For this review, take the finished solid that the model builds, in its own axes (mm). A direction names the side the tool comes from. Round coordinates to 2 decimals unless told otherwise and drop trailing zeros. Order: outer loops, then holes, each group sorted by start corner. A loop starts at its lowest first (then second) coordinate and runs counter-clockwise, first axis right, second up. Notation, with made-up numbers: (-15, -31.5) -> (31, -31.5) arc R19 ccw to (31, 5.5) -> close; hole circle Ø7 at (35.25, 68.25). An arc over 180 degrees is marked (long way). Answer in a Markdown table with one row per item.
```python
from build123d import *

# Parameters (mm, degrees)
F0_W     = 15
F0_H     = 90
F0_R     = 1.5
F1_DEPTH = 3
F2_W     = 15
F2_H     = 3
F3_DEPTH = 18
F4_R     = 2.25
F5_DEPTH = 53.001


with BuildPart() as f1:
    # F0 (on Front) → F1 (new body)
    with BuildSketch(Plane.XZ):
        Rectangle(F0_W, F0_H)
        with Locations((0, -39)):
            Circle(F0_R, mode=Mode.SUBTRACT)
        with Locations((0, 41)):
            Circle(F0_R, mode=Mode.SUBTRACT)
    extrude(amount=F1_DEPTH)

    # F2 (on face) → F3 (join)
    with BuildSketch(Plane.XZ.offset(3)):
        with Locations((0, 6.5)):
            Rectangle(F2_W, F2_H)
    extrude(amount=F3_DEPTH)

    # F4 (on face) → F5 (cut, through all)
    with BuildSketch(Plane.XY.offset(8)):
        with Locations((0, -12)):
            Circle(F4_R)
    extrude(amount=-F5_DEPTH, mode=Mode.SUBTRACT)


solid = f1.part
```
Q1. To check wall thickness, follow probe 1 along Z at (x, y) = (0, -1.7); probe 2 along Y at (x, z) = (0, 7); probe 3 along Z at (x, y) = (1.5, -13.75). State the ranges of each line that lie inside material, in increasing order.
Answer key:
| item | result |
|---|---|
| probe 1 | z = -45 to -40.5, -37.5 to 39.5, 42.5 to 45 |
| probe 2 | y = -21 to -14.25, -9.75 to 0 |
| probe 3 | z = 5 to 8 |
Q2. Take a section at A-A, the plane x = 0. Write out the cut boundary in (y, z), then the cut area to 4 significant figures.
Answer key:
| item | result |
|---|---|
| outline | (-21, 5) -> (-14.25, 5) -> (-14.25, 8) -> (-21, 8) -> close; (-9.75, 5) -> (-3, 5) -> (-3, -37.5) -> (0, -37.5) -> (0, 39.5) -> (-3, 39.5) -> (-3, 8) -> (-9.75, 8) -> close; (-3, -45) -> (0, -45) -> (0, -40.5) -> (-3, -40.5) -> close; (-3, 42.5) -> (0, 42.5) -> (0, 45) -> (-3, 45) -> close |
| area | 292.5 mm^2 |
Q3. Clearance check with flat-ended pins moving along their axes: pin 1 Ø7.5 at (x, y) = (3, -16) entering from +Z; pin 2 Ø5 at (x, z) = (-5.5, -8.5) entering from +Y; pin 3 Ø3 at (x, y) = (-4, -16) entering from -Z; pin 4 Ø4.5 at (x, z) = (3.5, 32) entering from -Y. State where each tip first meets the part, or that it passes through.
Answer key:
| item | result |
|---|---|
| pin 1 | stops at z = 8 |
| pin 2 | stops at y = 0 |
| pin 3 | stops at z = 5 |
| pin 4 | stops at y = -3 |
Q4. Take a section at C-C, the plane y = -12. Write out the cut boundary in (x, z).
Answer key:
| item | result |
|---|---|
| outline | (-7.5, 5) -> (-2.25, 5) -> (-2.25, 8) -> (-7.5, 8) -> close; (2.25, 5) -> (7.5, 5) -> (7.5, 8) -> (2.25, 8) -> close |
Q5. Take a section at B-B, the plane z = 41. Write out the cut boundary in (x, y), then the cut area to 3 significant figures.
Answer key:
| item | result |
|---|---|
| outline | (-7.5, -3) -> (-1.5, -3) -> (-1.5, 0) -> (-7.5, 0) -> close; (1.5, -3) -> (7.5, -3) -> (7.5, 0) -> (1.5, 0) -> close |
| area | 36.0 mm^2 |
Q6. The part is to be moulded in two halves that separate along Z. For faces 1 (the face through (-0.325, -1.479, 39.536)), 2 (the face through (-7.5, -2.7, -0.2)), 3 (the face through (-2, -14, 8)), say which applies: +Z half, -Z half, draft (parallel to the pull), parting line (faces both ways), or undercut.
Answer key:
| item | result |
|---|---|
| face 1 | undercut |
| face 2 | draft |
| face 3 | +Z half |
Q7. Take a section at D-D, the plane x = 6. Write out the cut boundary in (y, z).
Answer key:
| item | result |
|---|---|
| outline | (-21, 5) -> (-3, 5) -> (-3, -45) -> (0, -45) -> (0, 45) -> (-3, 45) -> (-3, 8) -> (-21, 8) -> close |
Q8. Tool access review of faces 4 (the face through (0, -3, 27)), 5 (the face through (-2, -14, 5)), 6 (the face through (0, 0, 1)): name each direction out of +Z, -Z, +X, -X, +Y, -Y from which nothing blocks a thin tool from reaching the whole face with its end or side.
Answer key:
| item | result |
|---|---|
| face 4 | +Z, +X, -X, -Y |
| face 5 | -Z, +X, -X, -Y |
| face 6 | +Z, -Z, +X, -X, +Y |
